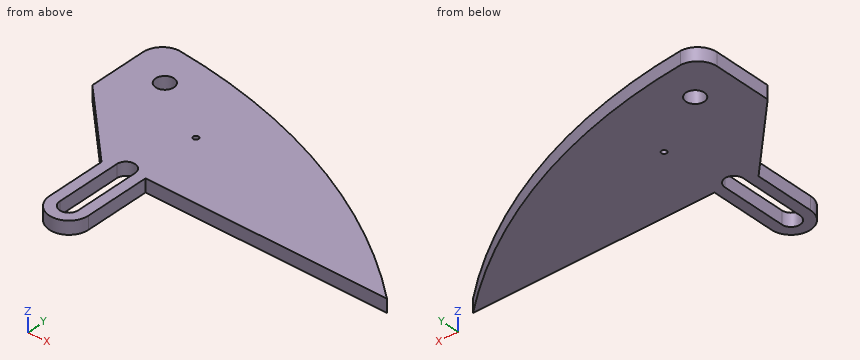
Autodesk Inventor part; units mm, degrees
ref_plane "YZ Plane" through (0, 0, 0) normal (1, 0, 0) x (0, 1, 0)
ref_plane "XZ Plane" through (0, 0, 0) normal (0, 1, 0) x (-1, 0, 0)
ref_plane "XY Plane" through (0, 0, 0) normal (0, 0, 1) x (1, 0, 0)
sketch "Sketch1" plane through (0, 0, 0) normal (0, 0, 1) x (1, 0, 0)
  line L0 (7.5, 0) -> (7.5, -25)
  line L1 (0, -32.5) -> (0, -32.5)
  line L2 (-7.5, -25) -> (-7.5, -2.139)
  line L3 (0, 0) -> (0, -25) construction
  arc A0 (-7.5, -25) -> (0, -32.5) centre (0, -25) ccw
  arc A1 (0, -32.5) -> (7.5, -25) centre (0, -25) ccw
  line L4 (0, -28.5) -> (0, -28.5)
  line L5 (-3.5, -25) -> (-3.5, 0)
  line L6 (0, 3.5) -> (0, 3.5)
  line L7 (3.5, 0) -> (3.5, -25)
  arc A2 (-3.5, -25) -> (0, -28.5) centre (0, -25) ccw
  arc A3 (0, -28.5) -> (3.5, -25) centre (0, -25) ccw
  arc A4 (3.5, 0) -> (0, 3.5) centre (0, 0) ccw
  arc A5 (0, 3.5) -> (-3.5, 0) centre (0, 0) ccw
  line L8 (7.5, 0) -> (100, 0)
  line L9 (-35, 25.361) -> (-35, 47.5)
  line L10 (-7.5, -2.139) -> (-35, 25.361)
  line L11 (-7.5, -2.139) -> (31.3909, -2.139) construction
  arc A6 (-27.5, 55) -> (-35, 47.5) centre (-27.5, 47.5) ccw
  arc A7 (100, 0) -> (-27.5, 55) centre (-45.2542, -161.4415) ccw
  point P0 (0, 0)
  point P1 (-20, 40)
  point P2 (0, -28.5)
  point P3 (0, 3.5)
  point P4 (0, -32.5)
  dimension "d0" = 20
  dimension "d2" = 25
  dimension "d8" = 15
  dimension "d9" = 7.5
  dimension "d10" = 7.5
  dimension "d11" = 3.5
  dimension "d12" = 3.5
  dimension "d13" = 7
  dimension "d14" = 3.5
  dimension "d28" = 40
  dimension "d30" = 135
  dimension "d31" = 15
  dimension "d33" = 7.5
  dimension "d34" = 120
  dimension "d35" = 217.1685
  dimension "d36" = 27.5
extrude "Extrusion1" add sketch "Sketch1" along normal blind 5
sketch "Sketch3" plane through (0, 0, 5) normal (0, 0, 1) x (1, 0, 0)
  arc A0 (-27.7773, 74.9035) -> (-35, 67.9071) centre (-28, 67.9071) ccw
  point P0 (0, 0)
  point P1 (-20, 40)
  dimension "d26" = 20
  dimension "d27" = 40
hole "Hole1" at (-20, 40, 5) direction (0, 0, -1) diameter 7 end through all
sketch "Sketch4" plane through (0, 0, 5) normal (0, 0, 1) x (1, 0, 0)
  line L0 (7.5, 0) -> (100, 0)
  line L1 (-35, 47.5) -> (-35, 25.361)
  circle A0 centre (5, 25) radius 20 construction
  point P0 (0, 0)
  dimension "d37" = 25
  dimension "d38" = 40
  dimension "d39" = 40
hole "Hole2" at (5, 25, 5) direction (0, 0, -1) diameter 2 end through all
properties part number "Dedo-BC" material "MDF Medium Density Fiberboard"
The model under review builds one solid part; all positions refer to its coordinate system, in mm. Round coordinates to 2 decimals unless told otherwise and drop trailing zeros. Order: outer loops, then holes, each group sorted by start corner. A loop starts at its lowest first (then second) coordinate and runs counter-clockwise, first axis right, second up.
(1) Wall thickness on L1, parallel to X at y = -6.5, z = 3.3; L2, parallel to X at y = 40, z = 3.95; L3, parallel to Y at x = -23, z = 2.8: over which ranges is each line inside the solid? List them lowest first.
Working result:
L1: x = -7.5 to -3.5, 3.5 to 7.5
L2: x = -35 to -23.5, -16.5 to 35.88
L3: y = 13.36 to 38.2, 41.8 to 54.58
(2) Take a section at A-A, the plane y = -22.5. State the section outline as (x, z) points.
Working result:
outline: (-7.5, 0) - (-3.5, 0) - (-3.5, 5) - (-7.5, 5) - close; (3.5, 0) - (7.5, 0) - (7.5, 5) - (3.5, 5) - close
(3) Take a section at D-D, the plane y = 17. State the section outline as (x, z) points.
Working result:
outline: (-26.64, 0) - (78.52, 0) - (78.52, 5) - (-26.64, 5) - close
(4) Take a section at C-C, the plane z = 1.6. State the section outline as (x, y) points.
Working result:
outline: (-35, 25.36) - (-7.5, -2.14) - (-7.5, -25) arc R7.5 ccw to (7.5, -25) - (7.5, 0) - (100, 0) arc R217.17 ccw to (-27.5, 55) arc R7.5 ccw to (-35, 47.5) - close; hole circle Ø7 at (-20, 40); hole (-3.5, -25) arc R3.5 ccw to (3.5, -25) - (3.5, 0) arc R3.5 ccw to (-3.5, 0) - close; hole circle Ø2 at (5, 25)
(5) For P1, Ø1, axis at x = -19.5, z = 0.5, coming from the -Y side; P2, Ø2.5, axis at y = -12.5, z = 2.5, coming from the -X side; P3, Ø2.5, axis at y = -10, z = 2, coming from the +X side, all flat-tipped, find the tip position at first contact; note any pin that passes through.
Working result:
P1: stops at y = 9.36
P2: stops at x = -7.5
P3: stops at x = 7.5
(6) Take a section at B-B, the plane x = -20. State the section outline as (y, z) points.
Working result:
outline: (10.36, 0) - (36.5, 0) - (36.5, 5) - (10.36, 5) - close; (43.5, 0) - (54.25, 0) - (54.25, 5) - (43.5, 5) - close
